Can you work these out from the drawing? Everything is in mm from the part's minimum corner. A direction names the side the tool comes from. Coordinates: 2 decimals unless noted, no trailing zeros. Order: outer loops, then holes, each group sorted by start corner. A loop starts at its lowest first (then second) coordinate and runs counter-clockwise, first axis right, second up. Notation, with made-up numbers: (-34, 32) - (24, 32) arc R14 cw to (24, 57) - close; hole circle Ø8 at (11, 68). An arc over 180 degrees is marked (long way). Answer as CSV lines item,"result". Start each with the question number.
Q1. For the marked faces 1 and 2, which set-ups out of +Z, -Z, +X, -X, +Y, -Y let a thin tool reach every point of the face, with its end or its side?
Q2. Suppose I cut it at B-B (y = 23). Please give me the cut outline in (x, z).
Q3. Suppose I cut it at A-A (x = 31). Please give me the cut outline in (y, z).
Q4. Suppose I cut it at C-C (x = 21). Please give me the cut outline in (y, z).
Q5. For pin 1 Ø8 at (x, y) = (12.5, 6.5) entering from +Z; pin 2 Ø1.5 at (x, y) = (8.5, 30.5) entering from -Z, each with a flat end and sliding along its axis, tell me the tip position at first contact or that it passes through.
Q6. I need wall thicknesses on line 1 (Y direction, x = 6, z = 0.85); line 2 (Y direction, x = 6, z = 1); line 3 (Z direction, x = 33.5, y = 21). Which ranges of each line are inside material? Lowest first, please.
Q7. Suppose I cut it at D-D (z = 18.5). Please give me the cut outline in (x, y).
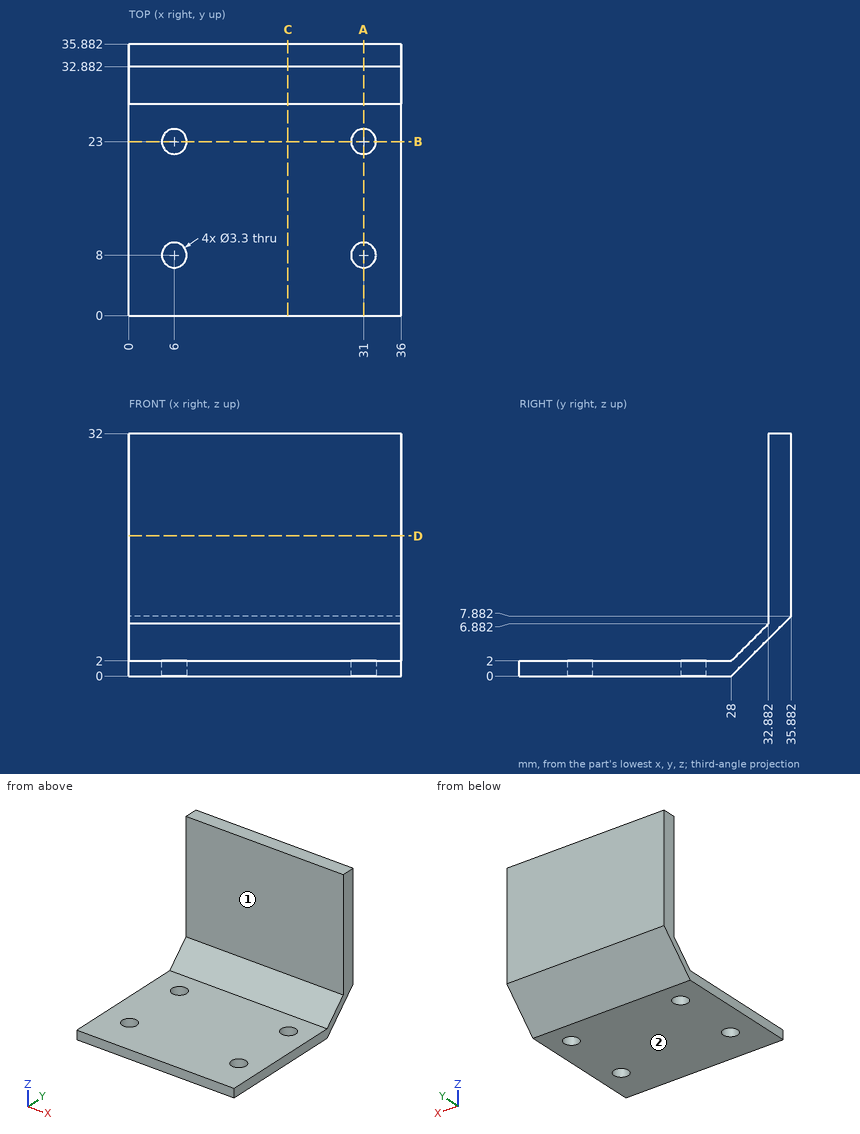
Here are the results:
1,face 1,"+Z, +X, -X, -Y"
1,face 2,"-Z, +X, -X, +Y, -Y"
2,outline,"(0, 0) - (4.35, 0) - (4.35, 2) - (0, 2) - close; (7.65, 0) - (29.35, 0) - (29.35, 2) - (7.65, 2) - close; (32.65, 0) - (36, 0) - (36, 2) - (32.65, 2) - close"
3,outline,"(0, 0) - (6.35, 0) - (6.35, 2) - (0, 2) - close; (9.65, 0) - (21.35, 0) - (21.35, 2) - (9.65, 2) - close; (24.65, 0) - (28, 0) - (35.88, 7.88) - (35.88, 32) - (32.88, 32) - (32.88, 6.88) - (28, 2) - (24.65, 2) - close"
4,outline,"(0, 0) - (28, 0) - (35.88, 7.88) - (35.88, 32) - (32.88, 32) - (32.88, 6.88) - (28, 2) - (0, 2) - close"
5,pin 1,"stops at z = 2"
5,pin 2,"stops at z = 1.75"
6,line 1,"y = 0 to 6.35, 9.65 to 21.35, 24.65 to 28.85"
6,line 2,"y = 0 to 6.35, 9.65 to 21.35, 24.65 to 29"
6,line 3,"z = 0 to 2"
7,outline,"(0, 32.88) - (36, 32.88) - (36, 35.88) - (0, 35.88) - close"
